from build123d import *

# Parameters (mm, degrees)
F0_R     = 12.7
F1_DEPTH = 6.35
F2_R     = 8.063613
F3_DEPTH = 0.762
F4_R     = 7.9375
F5_DEPTH = 68.58
F6_R     = 6.35
F7_DEPTH = 12.7
F9_DEPTH = 6.35


with BuildPart() as f1:
    # F0 (on Right) → F1 (new body, symmetric)
    with BuildSketch(Plane.YZ):
        Circle(F0_R)
    extrude(amount=F1_DEPTH, both=True)

    # F2 (on face) → F3 (join)
    with BuildSketch(Plane.YZ.offset(6.35)):
        Circle(F2_R)
    extrude(amount=F3_DEPTH)

    # F4 (on face) → F5 (join)
    with BuildSketch(Plane.YZ.offset(7.112)):
        Circle(F4_R)
    extrude(amount=F5_DEPTH)

    # F6 (on face) → F7 (join)
    with BuildSketch(Plane.YZ.offset(75.692)):
        Circle(F6_R)
    extrude(amount=F7_DEPTH)

    # F8 (on face) → F9 (cut)
    with BuildSketch(Plane(origin=(-6.35, 0, 0), x_dir=(0, -1, 0), z_dir=(-1, 0, 0))):
        Polygon((6.555755, -3.784967), (6.555755, 3.784967), (0, 7.569933), (-6.555755, 3.784967), (-6.555755, -3.784967), (0, -7.569933), align=None)
    extrude(amount=-F9_DEPTH, mode=Mode.SUBTRACT)


solid = f1.part
For this review, take the finished solid that the model builds, in its own axes (mm). A direction names the side the tool comes from. Give positions to 0.01 mm unless a question says otherwise; leave off trailing zeros. Loops run counter-clockwise (first coordinate to the right, second up) from the corner with the lowest first, then second, coordinate; pieces in that order, holes last. Notation, with made-up numbers: (-39.75, 14) - (-26.75, 14) arc R17 cw to (-26.75, 23) - close; hole circle Ø5 at (20, 58.5). An arc over 180 degrees is marked (long way). Write each question's results on one line, items separated by ' | '.
(1) Take a section at B-B (y = 1). Give the boundary of the cut face in (x, z).
Conclusion:
outline: (-6.35, -12.66) - (6.35, -12.66) - (6.35, -8) - (7.11, -8) - (7.11, -7.87) - (75.69, -7.87) - (75.69, -6.27) - (88.39, -6.27) - (88.39, 6.27) - (75.69, 6.27) - (75.69, 7.87) - (7.11, 7.87) - (7.11, 8) - (6.35, 8) - (6.35, 12.66) - (-6.35, 12.66) - (-6.35, 6.99) - (0, 6.99) - (0, -6.99) - (-6.35, -6.99) - close
(2) For faces 4 (the flat face through (0, 0, 0)), 5 (the cylindrical face through (40.92, -1.72, -7.75)), 6 (the flat face through (-6.35, 5, -5)), list the 3-axis set-ups (+Z, -Z, +X, -X, +Y, -Y) from which the entire face can be reached by the end or side of a thin tool; tool diameter is ignored.
Conclusion:
face 4: -X | face 5: +X | face 6: +Z, -Z, -X, +Y, -Y
(3) For line 1 along Y through (x, z) = (17.5, 0.5); line 2 along X through (y, z) = (10.5, -6.5); line 3 along X through (y, z) = (3.5, -3.75), list the stretches that pass through material, from the lowest coordinate up.
Conclusion:
line 1: -7.92 to 7.92 | line 2: -6.35 to 6.35 | line 3: 0 to 88.39
(4) Take a section at A-A (z = 0). Give the boundary of the cut face in (x, y).
Conclusion:
outline: (-6.35, -12.7) - (6.35, -12.7) - (6.35, -8.06) - (7.11, -8.06) - (7.11, -7.94) - (75.69, -7.94) - (75.69, -6.35) - (88.39, -6.35) - (88.39, 6.35) - (75.69, 6.35) - (75.69, 7.94) - (7.11, 7.94) - (7.11, 8.06) - (6.35, 8.06) - (6.35, 12.7) - (-6.35, 12.7) - (-6.35, 6.56) - (0, 6.56) - (0, -6.56) - (-6.35, -6.56) - close
(5) For pin 1 Ø1 at (x, y) = (32.5, -6.5) entering from -Z; pin 2 Ø1 at (x, z) = (30.5, -3.5) entering from +Y; pin 3 Ø3 at (x, y) = (51.5, -2) entering from -Z, all flat-tipped, find the tip position at first contact; note any pin that passes through.
Conclusion:
pin 1: z = -5.2 | pin 2: y = 7.35 | pin 3: z = -7.92
(6) Take a section at C-C (x = 12.5). Give the boundary of the cut face in (y, z) (1 decimal).
Conclusion:
outline: circle Ø15.9 at (0, 0)
(7) Draft analysis for pull direction Y (two halves, no side actions). For faces 1 (the flat face through (88.392, 0, 0)), 2 (the flat face through (-3, -6.556, 0)), 3 (the cylindrical face through (6.7, 7.7, 2.4)), state which applies: +Y half, -Y half, draft (parallel to the pull), parting line (faces both ways), or undercut.
Conclusion:
face 1: draft | face 2: undercut | face 3: parting line
